from build123d import *

# Parameters (mm, degrees)
SKETCH1_W           = 152.4
SKETCH1_H           = 81.28
BOSS_EXTRUDE1_DEPTH = 3.175
SKETCH2_R           = 3.175
SKETCH2_R_2         = 6.35
CUT_EXTRUDE1_DEPTH  = 173.74917952
CHAMFER1_SIZE       = 38.1
CHAMFER1_SIZE2      = 94.300809115
CHAMFER2_SIZE       = 127
CHAMFER2_SIZE2      = 22.39352655
CUT_EXTRUDE2_DEPTH  = 173.74917952
FILLET1_R           = 5.08
CUT_EXTRUDE3_DEPTH  = 173.74917952
SKETCH5_R           = 2.5796875
CUT_EXTRUDE4_DEPTH  = 173.749179658
CIRPATTERN1_COUNT   = 5
CIRPATTERN1_ANGLE   = 20


with BuildPart() as part:
    # Sketch1 → Boss-Extrude1 (new body)
    with BuildSketch(Plane(origin=(0, 0, 0), x_dir=(1, 0, 0), z_dir=(0, 1, 0))):
        with Locations((76.2, 40.64)):
            Rectangle(SKETCH1_W, SKETCH1_H)
    extrude(amount=BOSS_EXTRUDE1_DEPTH)

    # Sketch2 → Cut-Extrude1 (cut, through all)
    with BuildSketch(Plane(origin=(0, 3.175, 0), x_dir=(1, 0, 0), z_dir=(0, 1, 0))):
        with Locations(Location((12.7, 45.72, 0), (0, 0, 270))):
            Circle(SKETCH2_R)
        with Locations(Location((139.7, 63.5, 0), (0, 0, 270))):
            Circle(SKETCH2_R_2)
        with BuildLine():
            ThreePointArc((118.11, 45.72), (114.3, 49.53), (110.49, 45.72))
            ThreePointArc((110.49, 45.72), (109.15371332, 29.608970028), (105.181373622, 13.93825))
            ThreePointArc((105.181373622, 13.93825), (107.546294022, 9.096829599), (112.387714423, 11.46175))
            ThreePointArc((112.387714423, 11.46175), (116.669587085, 28.353565095), (118.11, 45.72))
        make_face()
    extrude(amount=-CUT_EXTRUDE1_DEPTH, mode=Mode.SUBTRACT)

    # Chamfer1
    chamfer1_edges = [part.edges().sort_by_distance(p)[0] for p in [
        (0, 1.5875, 0),
    ]]
    chamfer1_side = [part.faces().sort_by_distance(p)[0] for p in [
        (0, 1.5875, -40.64),
    ]]
    chamfer(chamfer1_edges, length=CHAMFER1_SIZE, length2=CHAMFER1_SIZE2, reference=chamfer1_side[0])

    # Chamfer2
    chamfer2_edges = [part.edges().sort_by_distance(p)[0] for p in [
        (0, 1.5875, -81.28),
    ]]
    chamfer2_side = [part.faces().sort_by_distance(p)[0] for p in [
        (76.2, 1.5875, -81.28),
    ]]
    chamfer(chamfer2_edges, length=CHAMFER2_SIZE, length2=CHAMFER2_SIZE2, reference=chamfer2_side[0])

    # Sketch3 → Cut-Extrude2 (cut, through all)
    with BuildSketch(Plane(origin=(0, 3.175, 0), x_dir=(1, 0, 0), z_dir=(0, 1, 0))):
        Polygon((134.62, 38.1), (129.54, 0), (152.4, 0), (152.4, 38.1), align=None)
    extrude(amount=-CUT_EXTRUDE2_DEPTH, mode=Mode.SUBTRACT)

    # Fillet1
    fillet1_edges = [part.edges().sort_by_distance(p)[0] for p in [
        (94.300809115, 1.5875, 0),
        (0, 1.5875, -38.1),
        (0, 1.5875, -58.88647345),
        (127, 1.5875, -81.28),
        (152.4, 1.5875, -38.1),
        (129.54, 1.5875, 0),
        (134.62, 1.5875, -38.1),
        (152.4, 1.5875, -81.28),
    ]]
    fillet(fillet1_edges, radius=FILLET1_R)

    # Sketch4 → Cut-Extrude3 (cut, through all)
    with BuildSketch(Plane(origin=(0, 3.175, 0), x_dir=(1, 0, 0), z_dir=(0, 1, 0))):
        with BuildLine():
            Line((79.02824603, 33.454322708), (63.267898808, 33.454322708))
            Line((63.267898808, 33.454322708), (63.267898808, 34.367135208))
            Line((63.267898808, 34.367135208), (70.958454364, 43.415885208))
            Line((70.958454364, 43.415885208), (63.267898808, 52.892378263))
            Line((63.267898808, 52.892378263), (63.267898808, 53.774322708))
            Line((63.267898808, 53.774322708), (78.768072419, 53.774322708))
            Line((78.768072419, 53.774322708), (79.072343253, 48.129878263))
            Line((79.072343253, 48.129878263), (77.687690475, 48.129878263))
            add(Edge.make_bspline(
                [(77.687690475, 48.129878263), (77.666267335, 48.312443932), (77.624982011, 48.664272977), (77.531920072, 49.166102178), (77.421008935, 49.62371596), (77.297338484, 50.038468153), (77.145364304, 50.406140244), (76.981241456, 50.731622206), (76.788125584, 51.007791949), (76.57914231, 51.245843364), (76.346452552, 51.448106373), (76.086781148, 51.614145073), (75.807782072, 51.761949969), (75.502009403, 51.881996436), (75.169445928, 51.96657961), (74.814820872, 52.034378559), (74.435667298, 52.073714003), (74.174700115, 52.078522896), (74.040850197, 52.080989374)],
                knots=[0, 0, 0, 0, 1.445989141, 2.78661909, 4.012434194, 5.150135165, 6.187474348, 7.139280037, 8.011906442, 8.831168962, 9.626489899, 10.428426412, 11.250947746, 12.10787495, 13.005585407, 13.946934481, 14.94698387, 16, 16, 16, 16], degree=3))
            Line((74.040850197, 52.080989374), (67.43949603, 52.080989374))
            Line((67.43949603, 52.080989374), (73.921787697, 44.280190763))
            Line((73.921787697, 44.280190763), (66.950016864, 36.27654493))
            Line((66.950016864, 36.27654493), (74.212829364, 36.27654493))
            add(Edge.make_bspline(
                [(74.212829364, 36.27654493), (74.36279346, 36.279802671), (74.654213785, 36.286133332), (75.077264171, 36.314305601), (75.470658519, 36.371763784), (75.832477573, 36.452086018), (76.16654489, 36.545672831), (76.468216936, 36.671559846), (76.742753798, 36.815646486), (76.99291299, 36.987221798), (77.223304318, 37.196939313), (77.442312889, 37.449316269), (77.65608094, 37.749183515), (77.859903069, 38.097852765), (78.063918522, 38.491956646), (78.259688528, 38.933240259), (78.457090359, 39.41997208), (78.571649199, 39.765370609), (78.63137103, 39.945433819)],
                knots=[0, 0, 0, 0, 1.136055194, 2.207658906, 3.209008574, 4.143648749, 5.013803629, 5.832513146, 6.614441668, 7.358687952, 8.123305807, 8.967432535, 9.885009082, 10.908395979, 12.023751854, 13.244578613, 14.563543328, 16, 16, 16, 16], degree=3))
            Line((78.63137103, 39.945433819), (79.919009919, 39.469183819))
            Line((79.919009919, 39.469183819), (79.02824603, 33.454322708))
        make_face()
    extrude(amount=-CUT_EXTRUDE3_DEPTH, mode=Mode.SUBTRACT)

    # Sketch5 → Cut-Extrude4 (cut, through all)
    with BuildSketch(Plane(origin=(0, 3.175, 0), x_dir=(1, 0, 0), z_dir=(0, 1, 0))):
        with Locations(Location((101.6, 45.72, 0), (0, 0, 270))):
            Circle(SKETCH5_R)
        with Locations(Location((93.912900428, 42.418, 0), (0, 0, 270))):
            Circle(SKETCH5_R)
    cut_extrude4 = extrude(amount=-CUT_EXTRUDE4_DEPTH, mode=Mode.SUBTRACT)

    # CirPattern1: Cut-Extrude4 ×5 about axis
    cirpattern1_axis = Axis((12.7, 0, -45.72), (0, -1, 0))
    for i in range(1, CIRPATTERN1_COUNT):
        add(cut_extrude4.rotate(cirpattern1_axis, i * CIRPATTERN1_ANGLE / (CIRPATTERN1_COUNT - 1)), mode=Mode.SUBTRACT)


solid = part.part
The listing builds one solid part. Answer for the finished solid, in the listing's coordinates (mm). A direction names the side the tool comes from. Give positions to 0.01 mm unless a question says otherwise; leave off trailing zeros. Write each loop counter-clockwise with the first axis right and the second up, starting at its lowest first coordinate (ties: lowest second). Pieces come first, ordered by that corner, then holes.
Item 1: Section A-A, the plane x = 12.7 is taken. Write down the section's boundary in (y, z) (3 decimals), plus the area to 3 significant figures.
Item 2: Section C-C, the plane y = 2.6 is taken. Count the separate pieces of the cut face and the enclosed holes in it, plus the area to 3 significant figures.
Item 3: Determine the mould class of faces 3 (the flat face through (75, 0, -41)), 4 (the flat face through (152.4, 2, -59)), 5 (the cylindrical face through (90.174, 1.61, -16.031)) for opening direction X: released by +X, released by -X, zero draft, split by the parting line, or undercut.
Item 4: Flat-ended cylindrical pins translate along their axes: P1, Ø1, axis at x = 71.5, y = 1.5, coming from the +Z side; P2, Ø1, axis at x = 143.5, y = 2, coming from the +Z side; P3, Ø1.5, axis at x = 78, y = 1, coming from the -Z side. Find the tip coordinate at first contact, or state that the pin passes through.
Item 5: Find the intervals of material crossed by line 1 along X through (y, z) = (0.3, -15); line 2 along X through (y, z) = (2.2, -22); line 3 along X through (y, z) = (0.85, -45.5), in increasing order.
Item 6: Section B-B, the plane z = -63.5 is taken. Write down the section's boundary in (x, y) (3 decimals), plus the area to 3 significant figures.
Item 7: Which of the six approach directions +Z, -Z, +X, -X, +Y, -Y give full straight-line access (tool end or side, diameter ignored) to faces 1 (the flat face through (71, 2, -52.081)), 2 (the cylindrical face through (135.76, 1.565, -36.876))?
Item 8: Section D-D, the plane x = 50.5 is taken. Write down the section's boundary in (y, z) (3 decimals), plus the area to 3 significant figures.
Completed:
1. outline: (0, -61.126) - (3.175, -61.126) - (3.175, -48.895) - (0, -48.895) - close; (0, -42.545) - (3.175, -42.545) - (3.175, -32.969) - (0, -32.969) - close
1. area: 69.2 mm2
2. separate pieces: 1
2. enclosed holes: 14
2. area: 7,580 mm2
3. face 3: zero draft
3. face 4: released by +X
3. face 5: undercut
4. P1: stops at z = -9.01
4. P2: stops at z = -38.1
4. P3: stops at z = -72.77
5. line 1: x = 57.17 to 85.31, 90.46 to 93.68, 98.8 to 105.54, 113.53 to 131.54
5. line 2: x = 39.85 to 87.76, 92.82 to 96.09, 101.05 to 107.57, 115.41 to 132.47
5. line 3: x = 0 to 9.53, 15.87 to 69.27, 72.91 to 99.03, 104.17 to 110.49, 118.11 to 152.4
6. outline: (26.165, 0) - (133.35, 0) - (133.35, 3.175) - (26.165, 3.175) - close; (146.05, 0) - (152.4, 0) - (152.4, 3.175) - (146.05, 3.175) - close
6. area: 360 mm2
7. face 1: +Y, -Y
7. face 2: +Z, +X, +Y, -Y
8. outline: (0, -67.791) - (3.175, -67.791) - (3.175, -17.697) - (0, -17.697) - close
8. area: 159 mm2
